from build123d import *

# Parameters (mm, degrees)
BOSS_EXTRU_2_DEPTH      = 3
ENL_V_MAT_EXTRU_1_DEPTH = 141.768934672
EMPREINTE1_START        = 63.105178129
EMPREINTE1_DEPTH        = 3
EMPREINTE1_START_2      = 93.105178129
EMPREINTE1_2_DEPTH      = 3
BOSS_EXTRU_3_DEPTH      = 3


# Read off the part's stored shape, not the designer's step: Empreinte1
with BuildPart() as part:
    # Esquisse1 → Boss.-Extru.2 (new body)
    with BuildSketch(Plane.XY):
        with BuildLine():
            Line((40.247233076, 111.105178129), (40.247233076, 61.105178129))
            ThreePointArc((40.247233076, 61.105178129), (44.191308202, 49.180108885), (54.467960723, 41.95837654))
            add(Edge.make_bspline(
                [(54.467960723, 41.95837654), (93.469157599, 30.186251687), (94.060386504, -42.130931626), (70.625681641, -69.023414216)],
                knots=[0.073601613, 0.073601613, 0.073601613, 0.073601613, 1, 1, 1, 1], degree=3))
            Line((70.625681641, -69.023414216), (63.086562616, -62.453658944))
            add(Edge.make_bspline(
                [(51.578324546, 32.384975746), (52.441823747, 32.124337068), (54.160244695, 31.504173294), (57.306848095, 29.97035453), (60.909260152, 27.464002891), (64.778911343, 23.487842732), (69.333722485, 16.888912111), (73.713189985, 6.383804922), (76.439302823, -8.617528818), (76.523407917, -21.892716717), (75.336804817, -32.248132674), (73.851279993, -39.698340102), (71.811754469, -46.646923176), (69.699842941, -51.863805262), (67.806756273, -55.601272185), (66.298875889, -58.166006571), (64.985680603, -60.08494816), (63.904092742, -61.488799964), (63.366023798, -62.13296342), (63.086562616, -62.453658944)],
                knots=[0.073601613, 0.073601613, 0.073601613, 0.073601613, 0.102551563, 0.131501512, 0.189401411, 0.247301311, 0.30520121, 0.421001008, 0.536800806, 0.652600605, 0.710500504, 0.768400403, 0.826300302, 0.884200202, 0.913150151, 0.942100101, 0.97105005, 0.985525025, 1, 1, 1, 1], degree=3))
            ThreePointArc((51.578324546, 32.384975746), (36.163345766, 43.217574263), (30.247233076, 61.105178129))
            Line((30.247233076, 61.105178129), (30.247233076, 111.105178129))
            Line((30.247233076, 111.105178129), (40.247233076, 111.105178129))
        make_face()
    extrude(amount=BOSS_EXTRU_2_DEPTH)

    # Esquisse2 → Enlèv. mat.-Extru.1 (cut, through all)
    with BuildSketch(Plane.XY.offset(3)):
        with BuildLine():
            Line((58.604840791, -65.718091867), (72.675095618, -21.396789164))
            Line((72.675095618, -21.396789164), (77.883188433, -27.569343611))
            ThreePointArc((77.883188433, -27.569343611), (79.106345528, -28.256142913), (80.479757382, -27.970579539))
            Line((80.479757382, -27.970579539), (87.91787168, -23.272823141))
            Line((87.91787168, -23.272823141), (76.157367596, -75.355055511))
            Line((76.157367596, -75.355055511), (58.604840791, -65.718091867))
        make_face()
    extrude(amount=-ENL_V_MAT_EXTRU_1_DEPTH, mode=Mode.SUBTRACT)

    # Empreinte1 outline → Empreinte1 (cut)
    with BuildSketch(Plane(origin=(0, 0, 0), x_dir=(1, 0, 0), z_dir=(0, 1, 0)).offset(EMPREINTE1_START)):
        with BuildLine():
            ThreePointArc((40.222725568, -0.2), (40.219098005, -0.099995306), (40.215220265, 0))
            Line((40.215220265, 0), (30.247233076, 0))
            Line((30.247233076, 0), (30.247233076, -3))
            Line((30.247233076, -3), (35.247233076, -3))
            Line((35.247233076, -3), (35.247233076, -0.2))
            Line((35.247233076, -0.2), (40.222725568, -0.2))
        make_face()
    extrude(amount=EMPREINTE1_DEPTH, mode=Mode.SUBTRACT)

    # Empreinte1 2 outline → Empreinte1 2 (cut)
    with BuildSketch(Plane(origin=(0, 0, 0), x_dir=(1, 0, 0), z_dir=(0, 1, 0)).offset(EMPREINTE1_START_2)):
        with BuildLine():
            ThreePointArc((40.222725568, -0.2), (40.219098005, -0.099995306), (40.215220265, 0))
            Line((40.215220265, 0), (30.247233076, 0))
            Line((30.247233076, 0), (30.247233076, -3))
            Line((30.247233076, -3), (35.247233076, -3))
            Line((35.247233076, -3), (35.247233076, -0.2))
            Line((35.247233076, -0.2), (40.222725568, -0.2))
        make_face()
    extrude(amount=EMPREINTE1_2_DEPTH, mode=Mode.SUBTRACT)

    # Esquisse3 → Boss.-Extru.3 (add)
    with BuildSketch(Plane(origin=(0, 0, 0), x_dir=(-1, 0, 0), z_dir=(0, 0, -1))):
        with BuildLine():
            Line((-40.247233076, 111.105178129), (-30.247233076, 111.105178129))
            add(Edge.make_bspline(
                [(-30.247233076, 111.105178129), (-30.247233076, 112.14596965), (-30.217698493, 114.25472522), (-30.045014328, 118.252405482), (-29.624674548, 122.993020115), (-28.820656407, 128.236554261), (-27.74447291, 133.062686625), (-26.422917169, 137.485210513), (-24.367231012, 142.870966444), (-21.306772788, 148.697507946), (-17.00171943, 154.423085647), (-12.168743747, 159.053182078), (-6.886412749, 162.716784457), (0.639998699, 166.423733084), (8.67921262, 168.46569452), (16.603362122, 169.022509829), (22.293283685, 168.760231201), (27.526974489, 167.899846277), (31.325094184, 166.77680064), (33.908111954, 165.718326704), (35.589474071, 164.872941274), (36.748498996, 164.160369864), (37.530944286, 163.599193527), (37.852299425, 163.343502605), (38.016109762, 163.205698113)],
                knots=[0, 0, 0, 0, 0.015625, 0.03125, 0.0625, 0.09375, 0.125, 0.15625, 0.1875, 0.25, 0.3125, 0.375, 0.4375, 0.5, 0.625, 0.6875, 0.75, 0.8125, 0.875, 0.90625, 0.9375, 0.96875, 0.984375, 1, 1, 1, 1], degree=3))
            ThreePointArc((38.016109762, 163.205698113), (45.061039216, 163.813126294), (44.453611035, 170.858055748))
            add(Edge.make_bspline(
                [(-40.247233076, 111.105178129), (-40.247233076, 184.874305638), (25.539277275, 186.769628817), (44.453611035, 170.858055748)],
                knots=[0, 0, 0, 0, 1, 1, 1, 1], degree=3))
        make_face()
    extrude(amount=-BOSS_EXTRU_3_DEPTH)


solid = part.part
Work out the finished part from the listing and answer in its coordinate system (mm). Coordinates: 2 decimals unless noted, no trailing zeros. Write each loop counter-clockwise with the first axis right and the second up, starting at its lowest first coordinate (ties: lowest second). Pieces come first, ordered by that corner, then holes. Notation, with made-up numbers: M -40,69 L 8,69 A10 ccw 8,86 Z; hole C -35.5,51.25 d6. An arc over 180 degrees is marked long. Answer as CSV lines item,"result". Start each with the question number.
Item 1: Flat-ended cylindrical pins translate along their axes: P1, Ø0.9, axis at y = 75.5, z = 1.5, coming from the -X side; P2, Ø1.5, axis at x = 34.5, z = 1, coming from the +Y side; P3, Ø1.5, axis at y = 2.5, z = 2.5, coming from the -X side. Find the tip coordinate at first contact, or state that the pin passes through.
Item 2: Section A-A on y = 101 is taken. Write down the section's boundary in (x, z).
Item 3: Consider L1, parallel to X at y = 71, z = 1.6; L2, parallel to X at y = -20, z = 1.75; L3, parallel to Y at x = 4.5, z = 2.7. Determine where each line is inside the solid, lowest interval first.
Item 4: Section B-B on y = 48 is taken. Write down the section's boundary in (x, z).
Checks:
1,P1,"stops at x = 30.25"
1,P2,"stops at y = 146.07"
1,P3,"stops at x = 74.02"
2,outline,"M 30.25,0 L 40.25,0 L 40.25,3 L 30.25,3 Z"
3,L1,"x = 30.25 to 40.25"
3,L2,"x = 76.35 to 86.35"
3,L3,"y = 163.85 to 174.81"
4,outline,"M 33.26,0 L 45.14,0 L 45.14,3 L 33.26,3 Z"
